from build123d import *

# Parameters (mm, degrees)
ESBO_O1_W                = 41.5
ESBO_O1_H                = 22.5
RESSALTO_EXTRUS_O1_DEPTH = 3
ESBO_O2_W                = 9.25
ESBO_O2_H                = 22.5
RESSALTO_EXTRUS_O2_DEPTH = 3
ESBO_O3_W                = 6.5
ESBO_O3_H                = 22.5
RESSALTO_EXTRUS_O3_DEPTH = 3.25


with BuildPart() as part:
    # Esboço1 → Ressalto-extrusão1 (new body)
    with BuildSketch(Plane.XY):
        with Locations((4.5, 0)):
            Rectangle(ESBO_O1_W, ESBO_O1_H)
    extrude(amount=-RESSALTO_EXTRUS_O1_DEPTH)

    # Esboço2 → Ressalto-extrusão2 (add)
    with BuildSketch(Plane.ZY.offset(16.25)):
        with Locations((1.625, 0)):
            Rectangle(ESBO_O2_W, ESBO_O2_H)
    extrude(amount=RESSALTO_EXTRUS_O2_DEPTH)

    # Esboço3 → Ressalto-extrusão3 (add)
    with BuildSketch(Plane.XY.offset(-3)):
        with Locations((22, 0)):
            Rectangle(ESBO_O3_W, ESBO_O3_H)
    extrude(amount=RESSALTO_EXTRUS_O3_DEPTH)


solid = part.part
Work out the finished part from the listing and answer in its coordinate system (mm). A direction names the side the tool comes from. Give positions to 0.01 mm unless a question says otherwise; leave off trailing zeros. Write each loop counter-clockwise with the first axis right and the second up, starting at its lowest first coordinate (ties: lowest second). Pieces come first, ordered by that corner, then holes.
Q1. Given pin 1 (1.5 mm diameter, centred on x = -9, y = 6.5, fed in from +Z); pin 2 (3 mm diameter, centred on x = 23.5, y = 2.5, fed in from +Z), each flat-ended and moving along its own axis, determine where each tip first touches the part or whether it passes through.
Answer:
pin 1: stops at z = 0
pin 2: stops at z = 0.25
Q2. Straight lines are drawn through the part: L1, parallel to Z at x = 3.5, y = 0.5; L2, parallel to X at y = -7.75, z = 3.75; L3, parallel to Z at x = 22, y = 1.5. For each, find the intervals that lie inside material, in ascending order.
Answer:
L1: z = -3 to 0
L2: x = -19.25 to -16.25
L3: z = -3 to 0.25
Q3. The part is cut by section A-A on y = -5. Give the vertices of the cut face in (x, z), and give its area (3 significant figures).
Answer:
outline: (-19.25, -3) - (25.25, -3) - (25.25, 0.25) - (18.75, 0.25) - (18.75, 0) - (-16.25, 0) - (-16.25, 6.25) - (-19.25, 6.25) - close
area: 154 mm2
Q4. A tool of negligible diameter and unlimited length cuts with its end or side. For faces 1 (the face through (22, 0, 0.25)), 2 (the face through (1, 0, 0)), 3 (the face through (-19.25, 0, 2)), from which of +Z, -Z, +X, -X, +Y, -Y can it reach the whole face along a straight path? Write none if from no direction.
Answer:
face 1: +Z, +X, +Y, -Y
face 2: +Z, +Y, -Y
face 3: +Z, -Z, -X, +Y, -Y
Q5. The part is cut by section C-C on x = -8. Give the vertices of the cut face in (y, z).
Answer:
outline: (-11.25, -3) - (11.25, -3) - (11.25, 0) - (-11.25, 0) - close
Q6. The part is cut by section B-B on z = 4.25. Give the vertices of the cut face in (x, y).
Answer:
outline: (-19.25, -11.25) - (-16.25, -11.25) - (-16.25, 11.25) - (-19.25, 11.25) - close
